Geometry: final body of the model. Coordinates: model frame, mm. A direction names the side the tool comes from. Give positions to 0.01 mm unless a question says otherwise; leave off trailing zeros. Order: outer loops, then holes, each group sorted by start corner. A loop starts at its lowest first (then second) coordinate and runs counter-clockwise, first axis right, second up. Notation, with made-up numbers: (24, 84.25) -> (77, 84.25) arc R19 cw to (77, 113.25) -> close; hole circle Ø10 at (79.5, 14.5). An arc over 180 degrees is marked (long way). Write item = value, one per line.
```python
from build123d import *

# Parameters (mm, degrees)
F1_DEPTH        = 2
F3_DEPTH        = 10
F5_DEPTH        = 10
F8_DEPTH        = 2.5
F9_R            = 1.2
F11_D           = 3.2
F11_DEPTH       = 4.5
F11_CSINK_D     = 6
F11_CSINK_ANGLE = 90
F11_TIP         = 0.9613769904


with BuildPart() as f1:
    # F0 (on Top) → F1 (new body)
    with BuildSketch(Plane.XY):
        with BuildLine():
            Line((9, 9.75), (-9, 9.75))
            ThreePointArc((-9, 9.75), (-18.75, 0), (-9, -9.75))
            Line((-9, -9.75), (9, -9.75))
            ThreePointArc((9, -9.75), (18.75, 0), (9, 9.75))
        make_face()
    extrude(amount=F1_DEPTH)

    # F2 (on face) → F3 (join)
    with BuildSketch(Plane.XY.offset(2)):
        with BuildLine():
            Line((9, 9.75), (-9, 9.75))
            ThreePointArc((-9, 9.75), (-18.75, 0), (-9, -9.75))
            Line((-9, -9.75), (9, -9.75))
            ThreePointArc((9, -9.75), (18.75, 0), (9, 9.75))
        make_face()
        with BuildLine():
            ThreePointArc((9, 8.625), (17.625, 0), (9, -8.625))
            Line((9, -8.625), (-9, -8.625))
            ThreePointArc((-9, -8.625), (-17.625, 0), (-9, 8.625))
            Line((-9, 8.625), (9, 8.625))
        make_face(mode=Mode.SUBTRACT)
    extrude(amount=F3_DEPTH)

    # F4 (on face) → F5 (join)
    with BuildSketch(Plane.XY.offset(2)):
        with BuildLine():
            Line((2, 8.625), (-2, 8.625))
            ThreePointArc((-2, 8.625), (0, 6.625), (2, 8.625))
        make_face()
        with BuildLine():
            Line((-2, -8.625), (2, -8.625))
            ThreePointArc((2, -8.625), (0, -6.625), (-2, -8.625))
        make_face()
    extrude(amount=F5_DEPTH)

    # F7 (on offset) → F8 (join)
    with BuildSketch(Plane.XY.offset(9.5)):
        with BuildLine():
            ThreePointArc((2, 8.625), (0, 6.625), (-2, 8.625))
            Line((-2, 8.625), (-2, -8.625))
            ThreePointArc((-2, -8.625), (0, -6.625), (2, -8.625))
            Line((2, -8.625), (2, 8.625))
        make_face()
    extrude(amount=F8_DEPTH)

    # F9
    f9_edges = [f1.edges().sort_by_distance(p)[0] for p in [
        (2, 0, 12),
        (-2, 0, 12),
        (-2, 0, 9.5),
        (2, 0, 9.5),
    ]]
    fillet(f9_edges, radius=F9_R)

    # F11
    with Locations(Plane.XY.offset(2)):
        with Locations((-9, 0), (9, 0)):
            CounterSinkHole(F11_D / 2, F11_CSINK_D / 2, depth=F11_DEPTH, counter_sink_angle=F11_CSINK_ANGLE)
            with Locations((0, 0, -(F11_DEPTH + F11_TIP / 2))):  # 118° drill point
                Cone(0, F11_D / 2, F11_TIP, mode=Mode.SUBTRACT)


solid = f1.part
```
1) Mould query, pull axis X, two halves, no side actions, for faces 4 (the face through (0, 9.75, 6)), 5 (the face through (-18.748, 0.214, 5.916)), 6 (the face through (6, 8.625, 7)), 7 (the face through (17.623, 0.19, 6.93)). Classes: +X half, -X half, draft (parallel to the pull), parting line (faces both ways), or undercut.
Check sheet entries:
face_4 = draft
face_5 = -X half
face_6 = undercut
face_7 = undercut
2) Reachability of faces 1 (the face through (-6, -8.625, 7)), 2 (the face through (0, 0, 0)), 3 (the face through (-0.044, 6.625, 6.289)) from +Z, -Z, +X, -X, +Y, -Y: full face, straight path, thin tool, end or side. Return the list, or none.
Check sheet entries:
face_1 = +Z
face_2 = -Z, +X, -X, +Y, -Y
face_3 = none
3) Section query B-B (y = -5). Output: boundary loops of the cut face in (x, z), plus the area to 3 significant figures.
Check sheet entries:
outline = (-17.37, 0) -> (17.37, 0) -> (17.37, 12) -> (16.03, 12) -> (16.03, 2) -> (-16.03, 2) -> (-16.03, 12) -> (-17.37, 12) -> close; (-2, 10.7) arc R1.2 ccw to (-0.8, 9.5) -> (0.8, 9.5) arc R1.2 ccw to (2, 10.7) -> (2, 10.8) arc R1.2 ccw to (0.8, 12) -> (-0.8, 12) arc R1.2 ccw to (-2, 10.8) -> close
area = 105 mm²
4) Section query D-D (y = -8.25). Output: boundary loops of the cut face in (x, z), plus the area to 3 significant figures.
Check sheet entries:
outline = (-14.2, 0) -> (14.2, 0) -> (14.2, 12) -> (11.52, 12) -> (11.52, 2) -> (1.96, 2) -> (1.96, 10.41) arc R1.2 ccw to (2, 10.7) -> (2, 10.8) arc R1.2 ccw to (0.8, 12) -> (-0.8, 12) arc R1.2 ccw to (-2, 10.8) -> (-2, 10.7) arc R1.2 ccw to (-1.96, 10.41) -> (-1.96, 2) -> (-11.52, 2) -> (-11.52, 12) -> (-14.2, 12) -> close
area = 149 mm²
5) First-contact query: P1, Ø3, axis at y = -5, z = 10.5, coming from the -X side; P2, Ø1, axis at y = 5.5, z = 6, coming from the +X side; P3, Ø4, axis at y = -3, z = 3.5, coming from the +X side. Flat tips, straight axial feed; report the tip coordinate or a pass-through.
Check sheet entries:
P1 = -18.1
P2 = 17.37
P3 = 18.7
6) Line query: line 1 (X direction, y = 0, z = 0.1); line 2 (X direction, y = 0, z = 4.5) (3 decimals); line 3 (Y direction, x = -9, z = 0.35). Output: solid intervals per line, ascending. Write a range as from..to.
Check sheet entries:
line_1 = -18.75..-10.6, -7.4..7.4, 10.6..18.75
line_2 = -18.75..-17.625, 17.625..18.75
line_3 = -9.75..-1.6, 1.6..9.75
7) Section query C-C (x = 3.5). Output: boundary loops of the cut face in (y, z) (3 decimals).
Check sheet entries:
outline = (-9.75, 0) -> (9.75, 0) -> (9.75, 12) -> (8.625, 12) -> (8.625, 2) -> (-8.625, 2) -> (-8.625, 12) -> (-9.75, 12) -> close
8) Section query A-A (z = 8.5). Output: boundary loops of the cut face in (x, y) (3 decimals), plus the area to 3 significant figures.
Check sheet entries:
outline = (-9, -9.75) -> (9, -9.75) arc R9.75 ccw to (9, 9.75) -> (-9, 9.75) arc R9.75 ccw to start; hole (-9, -8.625) -> (-2, -8.625) arc R2 cw to (2, -8.625) -> (9, -8.625) arc R8.625 ccw to (9, 8.625) -> (2, 8.625) arc R2 cw to (-2, 8.625) -> (-9, 8.625) arc R8.625 ccw to start
area = 118 mm²
